Geometry check sheet. Reference: the model listing, model coordinates, mm. Face numbers are marked on the shaded views. A direction names the side the tool comes from. Give positions to 0.01 mm unless a question says otherwise; leave off trailing zeros. Loops run counter-clockwise (first coordinate to the right, second up) from the corner with the lowest first, then second, coordinate; pieces in that order, holes last. Notation, with made-up numbers: (69, 8) - (111, 8) arc R13 cw to (111, 13) - close; hole circle Ø1 at (42.25, -22). An arc over 180 degrees is marked (long way). Write item = value, one per line. Start each with the question number.
from build123d import *

# Parameters (mm, degrees)
CHAMFER1_SIZE      = 0.25
FILLET1_R          = 0.2
CUT_EXTRUDE1_DEPTH = 2
FILLET2_R          = 0.1


with BuildPart() as part:
    # Sketch1 → Revolve1 (revolve)
    with BuildSketch(Plane.XY):
        Polygon((0, -43), (-1.5, -43), (-1.5, -3), (-2.75, -3), (-2.75, 0), (0, 0), align=None)
    revolve(axis=Axis((0, 0, 0), (0, -1, 0)))

    # Chamfer1
    chamfer1_edges = [part.edges().sort_by_distance(p)[0] for p in [
        (1.5, -3, 0),
        (1.5, -43, 0),
    ]]
    chamfer(chamfer1_edges, length=CHAMFER1_SIZE)

    # Fillet1
    fillet1_edges = [part.edges().sort_by_distance(p)[0] for p in [
        (2.75, 0, 0),
    ]]
    fillet(fillet1_edges, radius=FILLET1_R)

    # Sketch2 → Cut-Extrude1 (cut)
    with BuildSketch(Plane(origin=(0, 0, 0), x_dir=(1, 0, 0), z_dir=(0, 1, 0))):
        Polygon((0, 1.443375673), (-1.25, 0.721687836), (-1.25, -0.721687836), (0, -1.443375673), (1.25, -0.721687836), (1.25, 0.721687836), align=None)
    extrude(amount=-CUT_EXTRUDE1_DEPTH, mode=Mode.SUBTRACT)

    # Fillet2
    fillet2_edges = [part.edges().sort_by_distance(p)[0] for p in [
        (0.625, -2, -1.082531755),
        (1.25, -2, 0),
        (0.625, -2, 1.082531755),
        (-0.625, -2, 1.082531755),
        (-1.25, -2, 0),
        (-0.625, -2, -1.082531755),
        (0.625, 0, -1.082531755),
        (-0.625, 0, -1.082531755),
        (-1.25, 0, 0),
        (-0.625, 0, 1.082531755),
        (0.625, 0, 1.082531755),
        (1.25, 0, 0),
    ]]
    fillet(fillet2_edges, radius=FILLET2_R)


solid = part.part
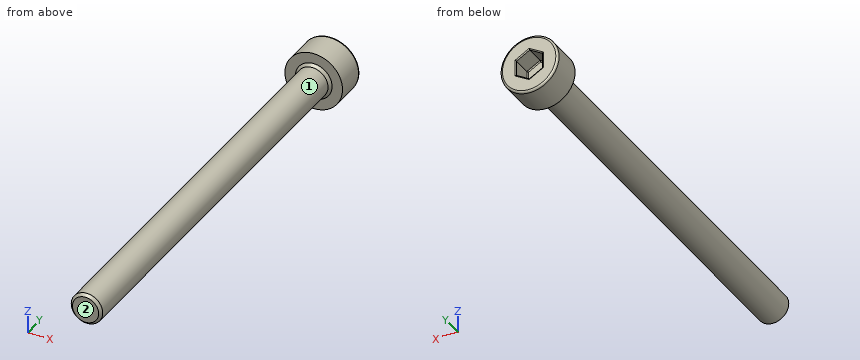
1) Tool access check on the marked faces 1 and 2. Record the directions out of +Z, -Z, +X, -X, +Y, -Y that give a thin tool (end or side, any length) a straight path to the whole face; none if there is none.
2) Gauge pin test, flat end, axial feed: P1, Ø1.8, axis at x = 0, z = 0, coming from the +Y side. Record the tip position at first contact, or that the pin passes through.
3) Cross-section at B-B on y = -36. Enter the section's corners in (x, z), and give its area (3 significant figures).
4) Material ranges on line 1 along Z through (x, y) = (0.2, -2.5); line 2 along Z through (x, y) = (0.65, -23.5); line 3 along Y through (x, z) = (-2.25, -1.1), recorded low to high.
5) Cross-section at A-A on z = 0. Enter the section's corners in (x, y), and give its area (3 significant figures).
Checked values:
q1.face_1 = -Y
q1.face_2 = +Z, -Z, +X, -X, -Y
q2.P1 = -2
q3.outline = circle Ø3 at (0, 0)
q3.area = 7.07 mm²
q4.line_1 = -2.74 to 2.74
q4.line_2 = -1.35 to 1.35
q4.line_3 = -3 to 0
q5.outline = (-2.75, -3) - (-1.75, -3) - (-1.5, -3.25) - (-1.5, -42.75) - (-1.25, -43) - (1.25, -43) - (1.5, -42.75) - (1.5, -3.25) - (1.75, -3) - (2.75, -3) - (2.75, -0.2) arc R0.2 ccw to (2.55, 0) - (1.35, 0) arc R0.1 ccw to (1.25, -0.1) - (1.25, -1.9) arc R0.1 cw to (1.15, -2) - (-1.15, -2) arc R0.1 cw to (-1.25, -1.9) - (-1.25, -0.1) arc R0.1 ccw to (-1.35, 0) - (-2.55, 0) arc R0.2 ccw to (-2.75, -0.2) - close
q5.area = 131 mm²
